Autodesk Inventor part; units mm, degrees
ref_plane "YZ Plane" through (0, 0, 0) normal (1, 0, 0) x (0, 1, 0)
ref_plane "XZ Plane" through (0, 0, 0) normal (0, 1, 0) x (-1, 0, 0)
ref_plane "XY Plane" through (0, 0, 0) normal (0, 0, 1) x (1, 0, 0)
sketch "Náčrt1" plane through (0, 0, 0) normal (0, 0, 1) x (1, 0, 0)
  line L0 (0, 15) -> (-3, 15)
  line L1 (-3, 15) -> (-3, 30)
  line L2 (-3, 30) -> (-6.6296, 30)
  line L3 (-7.3458, 29.8673) -> (-78.7162, 2.4924)
  line L4 (-80, 0.625) -> (-80, 0)
  line L5 (-80, 0) -> (0, 0)
  arc A0 (-78.7162, 2.4924) -> (-80, 0.625) centre (-78, 0.625) ccw
  arc A1 (-6.6296, 30) -> (-7.3458, 29.8673) centre (-6.6296, 28) ccw
  line L6 (0, 15) -> (0, 0)
  line L7 (0, 15) -> (3, 15)
  line L8 (3, 15) -> (3, 30)
  line L9 (3, 30) -> (6.6296, 30)
  line L10 (7.3458, 29.8673) -> (78.7162, 2.4924)
  line L11 (80, 0.625) -> (80, 0)
  line L12 (80, 0) -> (0, 0)
  arc A2 (80, 0.625) -> (78.7162, 2.4924) centre (78, 0.625) ccw
  arc A3 (7.3458, 29.8673) -> (6.6296, 30) centre (6.6296, 28) ccw
  point P0 (-7, 30)
  point P1 (-80, 2)
  point P2 (7, 30)
  point P3 (80, 2)
  dimension "d1" = 15
  dimension "d5" = 4
  dimension "d7" = 2
  dimension "d9" = 2
  dimension "d12" = 15
  dimension "d13" = 3
  dimension "d14" = 80
extrude "Vysunutí1" add sketch "Náčrt1" along normal mid plane 4
equation "\"d10\" = d4"
properties part number "LegLessMaterial"
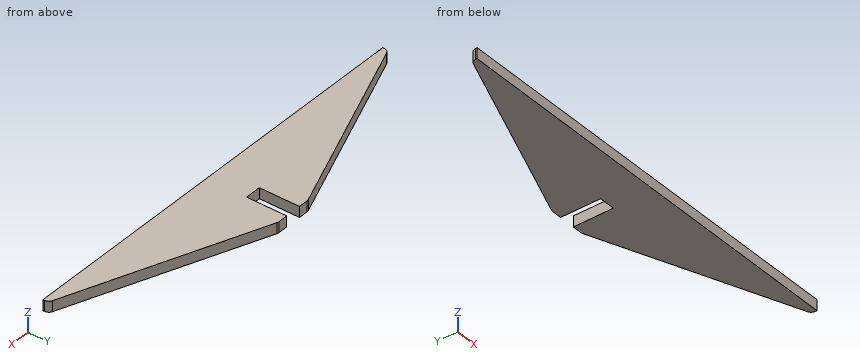
Read the model definition and answer for the solid it produces. Units are mm, in the model's axes. Round coordinates to 2 decimals unless told otherwise and drop trailing zeros. Order: outer loops, then holes, each group sorted by start corner. A loop starts at its lowest first (then second) coordinate and runs counter-clockwise, first axis right, second up.
1) The part is cut by section B-B on z = -1.25. Write down the section's boundary in (x, y) (3 decimals), plus the area to 3 significant figures.
2) The part is cut by section A-A on y = 22.5. Write down the section's boundary in (x, z).
3) The part is cut by section D-D on y = 8.5. Write down the section's boundary in (x, z), plus the area to 3 significant figures.
4) The part is cut by section C-C on x = 17.5. Write down the section's boundary in (y, z).
5) Flat-ended cylindrical pins translate along their axes: pin 1 (2 mm diameter, centred on x = 0, z = 0.5, fed in from +Y); pin 2 (1 mm diameter, centred on x = -7.5, z = 0, fed in from +Y). Find the tip coordinate at first contact, or state that the pin passes through.
6) Straight lines are drawn through the part: L1, parallel to Y at x = -1, z = -0.35; L2, parallel to Y at x = -49, z = 0. For each, find the intervals that lie inside material, in ascending order.
Resolved:
1. outline: (-80, 0) - (80, 0) - (80, 0.625) arc R2 ccw to (78.716, 2.492) - (7.346, 29.867) arc R2.002 ccw to (6.63, 30) - (3, 30) - (3, 15) - (-3, 15) - (-3, 30) - (-6.63, 30) arc R1.998 ccw to (-7.346, 29.867) - (-78.716, 2.492) arc R2 ccw to (-80, 0.625) - close
1. area: 2,670 mm2
2. outline: (-26.55, -2) - (-3, -2) - (-3, 2) - (-26.55, 2) - close; (3, -2) - (26.55, -2) - (26.55, 2) - (3, 2) - close
3. outline: (-63.05, -2) - (63.05, -2) - (63.05, 2) - (-63.05, 2) - close
3. area: 504 mm2
4. outline: (0, -2) - (25.97, -2) - (25.97, 2) - (0, 2) - close
5. pin 1: stops at y = 15
5. pin 2: stops at y = 29.97
6. L1: y = 0 to 15
6. L2: y = 0 to 13.89
